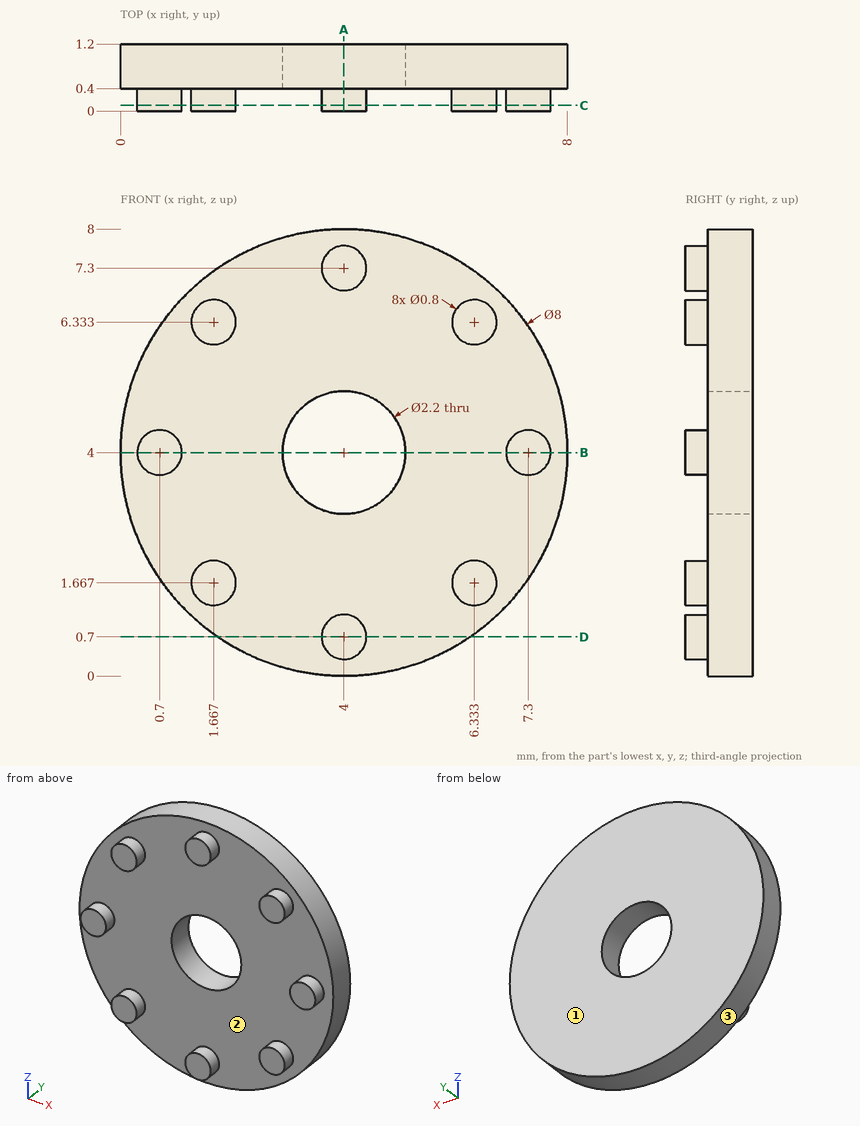
Verification items for this drawing (mm, ordinates from the low corner). Coordinates: 2 decimals unless noted, no trailing zeros. Write each loop counter-clockwise with the first axis right and the second up, starting at its lowest first coordinate (ties: lowest second). Pieces come first, ordered by that corner, then holes. Notation, with made-up numbers: M 24,86.25 L 74,86.25 A19 cw 74,109.25 Z; hole C 84.25,-6.5 d10. An arc over 180 degrees is marked long. One line per item, written item: value. Start each with the question number.
(1) Sectioned sample at D-D, the plane z = 0.7. Enter the section's corners in (x, y).
(2) Scan lines: line 1 along X through (y, z) = (0.85, 4); line 2 along Y through (x, z) = (3.25, 7). Record each from-to range of solid material in increasing order. Write a range as [from, to].
(3) Release check for a two-part mould opening along Z. For the marked faces 1, 2 and 3 record: released by +Z, released by -Z, zero draft, split by the parting line, or undercut.
(4) Sectioned sample at A-A, the plane x = 4. Enter the section's corners in (y, z).
(5) Depth check by flat-ended pin: pin 1 (1.5 mm diameter, centred on x = 4, z = 3.5, fed in from +Y). Enter the tip coordinate at first touch or a pass-through.
(6) Sectioned sample at C-C, the plane y = 0.1. Enter the section's corners in (x, z).
(7) Sectioned sample at B-B, the plane z = 4. Enter the section's corners in (x, y).
Filled sheet:
1. outline: M 1.74,0.4 L 3.6,0.4 L 3.6,0 L 4.4,0 L 4.4,0.4 L 6.26,0.4 L 6.26,1.2 L 1.74,1.2 Z
2. line 1: [0, 2.9], [5.1, 8]
2. line 2: [0.4, 1.2]
3. face 1: zero draft
3. face 2: undercut
3. face 3: split by the parting line
4. outline: M 0,0.3 L 0.4,0.3 L 0.4,0 L 1.2,0 L 1.2,2.9 L 0.4,2.9 L 0.4,1.1 L 0,1.1 Z; M 0,6.9 L 0.4,6.9 L 0.4,5.1 L 1.2,5.1 L 1.2,8 L 0.4,8 L 0.4,7.7 L 0,7.7 Z
5. pin 1: y = 1.2
6. outline: C 0.7,4 d0.8; C 1.67,1.67 d0.8; C 1.67,6.33 d0.8; C 4,0.7 d0.8; C 4,7.3 d0.8; C 6.33,1.67 d0.8; C 6.33,6.33 d0.8; C 7.3,4 d0.8
7. outline: M 0,0.4 L 0.3,0.4 L 0.3,0 L 1.1,0 L 1.1,0.4 L 2.9,0.4 L 2.9,1.2 L 0,1.2 Z; M 5.1,0.4 L 6.9,0.4 L 6.9,0 L 7.7,0 L 7.7,0.4 L 8,0.4 L 8,1.2 L 5.1,1.2 Z
